Can you work these out from the model? Positions are in its coordinate system, mm. A direction names the side the tool comes from. Round coordinates to 2 decimals unless told otherwise and drop trailing zeros. Order: outer loops, then holes, each group sorted by start corner. A loop starts at its lowest first (then second) coordinate and runs counter-clockwise, first axis right, second up. Notation, with made-up numbers: (-35.75, 57.5) -> (-21.75, 57.5) arc R9 ccw to (-21.75, 71.5) -> close; hole circle Ø10 at (15, 77.5). An arc over 180 degrees is marked (long way). One line per item, written item: value.
```python
from build123d import *

# Parameters (mm, degrees)
SKETCH1_R           = 7.5
BOSS_EXTRUDE1_DEPTH = 15
SKETCH1_3_R         = 5
BOSS_EXTRUDE2_DEPTH = 25
CUT_EXTRUDE1_DEPTH  = 42.382363393
SKETCH3_R           = 5
CUT_EXTRUDE2_DEPTH  = 15
CUT_EXTRUDE2_DRAFT  = -15
CIRPATTERN1_COUNT   = 18


with BuildPart() as part:
    # Sketch1 → Boss-Extrude1 (new body)
    with BuildSketch(Plane(origin=(0, 0, 0), x_dir=(1, 0, 0), z_dir=(0, 1, 0))):
        with Locations(Location((0, 0, 0), (0, 0, 270))):
            Circle(SKETCH1_R)
    extrude(amount=BOSS_EXTRUDE1_DEPTH)

    # Sketch1_3 → Boss-Extrude2 (add)
    with BuildSketch(Plane(origin=(0, 0, 0), x_dir=(1, 0, 0), z_dir=(0, 1, 0))):
        with Locations(Location((0, 0, 0), (0, 0, 270))):
            Circle(SKETCH1_3_R)
    extrude(amount=-BOSS_EXTRUDE2_DEPTH)

    # Sketch2 → Cut-Extrude1 (cut, through all)
    with BuildSketch(Plane(origin=(0, 15, 0), x_dir=(1, 0, 0), z_dir=(0, 1, 0))):
        with BuildLine():
            Line((1.572944175, 7.843841318), (1.13617114, 6.907178522))
            ThreePointArc((1.13617114, 6.907178522), (0.610090199, 6.973362887), (0.080508816, 6.999537008))
            Line((0.080508816, 6.999537008), (-0.186978867, 7.997814633))
            ThreePointArc((-0.186978867, 7.997814633), (0.697245942, 7.969557585), (1.572944175, 7.843841318))
        make_face()
    cut_extrude1 = extrude(amount=-CUT_EXTRUDE1_DEPTH, mode=Mode.SUBTRACT)


with BuildPart() as cut_extrude2_tool:
    # Sketch3 → Cut-Extrude2 (with draft: the straight prism first)
    with BuildSketch(Plane(origin=(0, 15, 0), x_dir=(1, 0, 0), z_dir=(0, 1, 0))):
        with Locations(Location((0, 0, 0), (0, 0, 270))):
            Circle(SKETCH3_R)
    extrude(amount=-CUT_EXTRUDE2_DEPTH)
    # Cut-Extrude2: the draft: its side faces are tilted about the plane it starts from
    cut_extrude2_sides = [cut_extrude2_tool.faces().sort_by_distance(p)[0] for p in [
        (0, 7.5, -5),
    ]]
    draft(cut_extrude2_sides, Plane(origin=(0, 15, 0), x_dir=(1, 0, 0), z_dir=(0, 1, 0)), CUT_EXTRUDE2_DRAFT)


with BuildPart() as part_1:
    add(part.part)

    # Cut-Extrude2: cut by cut_extrude2_tool
    add(cut_extrude2_tool.part, mode=Mode.SUBTRACT)

    # CirPattern1: Cut-Extrude1 ×18 about axis
    cirpattern1_axis = Axis((0, 0, 0), (0, 1, 0))
    for i in range(1, CIRPATTERN1_COUNT):
        add(cut_extrude1.rotate(cirpattern1_axis, i * 360 / CIRPATTERN1_COUNT), mode=Mode.SUBTRACT)


solid = part_1.part
```
Q1. I want a section at A-A on y = -15.5. List the corners of the cut face in (x, z) for me.
Answers below:
outline: circle Ø10 at (0, 0)
Q2. On a 3-axis mill with a long thin cutter (end or side, diameter ignored), from which of +Z, -Z, +X, -X, +Y, -Y can I reach the whole of each face in a straight line? I mean faces 1 (the face through (1.805, 7.605, 6.763)), 2 (the face through (-5, 0, 2)), 3 (the face through (-6.974, 7.605, 0.603)), 4 (the face through (6.15, 7.4, -4.29)). Say none if no direction works.
Answers below:
face 1: +Z, +Y, -Y
face 2: -Y
face 3: -X, +Y, -Y
face 4: -Z, +X, +Y, -Y
Q3. Please list where these lines run through material, in increasing order: line 1 along X through (y, z) = (-1, 0); line 2 along Y through (x, z) = (4.5, 2.75); line 3 along Z through (x, y) = (-5.5, 2).
Answers below:
line 1: -5 to 5
line 2: 0 to 15
line 3: -5.1 to -4.56, -4.33 to 4.65
Q4. We'd pull the mould along Z, two halves only. Please class faces 5 (the face through (-6.76, 7.6, -1.82)), 6 (the face through (6.76, 7.6, 1.82)), 7 (the face through (5.297, 7.395, 5.309)), 8 (the face through (-5, 15, 2)): released by +Z, released by -Z, zero draft, split by the parting line, or undercut.
Answers below:
face 5: undercut
face 6: undercut
face 7: released by +Z
face 8: zero draft
Q5. Will these pins go through, and if not, where does the flat tip stop? pin 1 Ø6 at (y, z) = (7, -6) entering from -X; pin 2 Ø2 at (y, z) = (-4.5, -5.5) entering from -X; pin 3 Ø8 at (x, y) = (5.5, 10) entering from +Z.
Answers below:
pin 1: x = -6.87
pin 2: x = -2.18
pin 3: z = 7.03
